Can you work these out from the model? Positions are in its coordinate system, mm. A direction names the side the tool comes from. Give positions to 0.01 mm unless a question says otherwise; leave off trailing zeros. Answer in a Markdown table with one row per item.
from build123d import *
from build123d.topology import SkipClean

# Parameters (mm, degrees)
SKETCH1_R           = 14.9
BOSS_EXTRUDE1_DEPTH = 2
SKETCH2_R           = 9.8
BOSS_EXTRUDE2_DEPTH = 8.5
SKETCH3_R           = 7.5
CUT_EXTRUDE1_DEPTH  = 5
THREAD1_PITCH       = 2
CUT_EXTRUDE2_START  = -3
SKETCH7_R           = 7.5
CUT_EXTRUDE2_DEPTH  = 3
SKETCH9_W           = 3.4
SKETCH9_H           = 17.333603835
BOSS_EXTRUDE3_DEPTH = 3
SKETCH10_R          = 0.75


with BuildPart() as part:
    # Sketch1 → Boss-Extrude1 (new body)
    with BuildSketch(Plane(origin=(0, 0, 0), x_dir=(1, 0, 0), z_dir=(0, 1, 0))):
        with Locations(Location((0, 0, 0), (0, 0, 270))):
            Circle(SKETCH1_R)
    extrude(amount=BOSS_EXTRUDE1_DEPTH)

    # Sketch2 → Boss-Extrude2 (add)
    with BuildSketch(Plane(origin=(0, 2, 0), x_dir=(1, 0, 0), z_dir=(0, 1, 0))):
        with Locations(Location((0, 0, 0), (0, 0, 270))):
            Circle(SKETCH2_R)
    extrude(amount=BOSS_EXTRUDE2_DEPTH)

    # Sketch3 → Cut-Extrude1 (cut)
    with BuildSketch(Plane(origin=(0, 10.5, 0), x_dir=(1, 0, 0), z_dir=(0, 1, 0))):
        with Locations(Location((0, 0, 0), (0, 0, 270))):
            Circle(SKETCH3_R)
    extrude(amount=-CUT_EXTRUDE1_DEPTH, mode=Mode.SUBTRACT)

    # Thread1: the profile of Sketch5 profile screwed along a right-hand helix of 5 turns, 10 arcs to a turn; built about Z, then put on its axis
    with SkipClean():  # the faces are left unmerged after this step: merging them gives an invalid solid
        thread1_z = Axis((0, 0, 0), (0, 0, 1))
        thread1_corners = [(9.8003, 0, -0.000173205), (9.8003, 0, 1.7501732), (8.71746825, 0, 1.124999997), (8.71746825, 0, 0.624999997)]
        with BuildLine(mode=Mode.PRIVATE) as thread1_profile:
            Line(thread1_corners[0], thread1_corners[1])
            Line(thread1_corners[1], thread1_corners[2])
            Line(thread1_corners[2], thread1_corners[3])
            Line(thread1_corners[3], thread1_corners[0])
        thread1_cap = Face(thread1_profile.wire())
        thread1_turn_angles = [0, 18, 36, 54, 72, 90, 108, 126, 144, 162, 180, 198, 216, 234, 252, 270, 288, 306, 324, 342, 360]
        thread1_turn_weights = [1, 0.9510565162951535, 1, 0.9510565162951535, 1, 0.9510565162951535, 1, 0.9510565162951535, 1, 0.9510565162951535, 1, 0.9510565162951535, 1, 0.9510565162951535, 1, 0.9510565162951535, 1, 0.9510565162951535, 1, 0.9510565162951535, 1]
        thread1_turn_rails = [Edge.make_bspline([Vector(p[0], p[1], 0).rotate(thread1_z, thread1_turn_angles[k]) / thread1_turn_weights[k] + Vector(0, 0, p[2] + THREAD1_PITCH * thread1_turn_angles[k] / 360) for k in range(21)], [0, 0, 0, 1, 1, 2, 2, 3, 3, 4, 4, 5, 5, 6, 6, 7, 7, 8, 8, 9, 9, 10, 10, 10], 2, thread1_turn_weights) for p in thread1_corners]
        thread1_turn_sides = [Face.make_surface_from_curves(thread1_turn_rails[p[0]], thread1_turn_rails[p[1]]) for p in [(0, 1), (1, 2), (2, 3), (3, 0)]]
        thread1 = Plane(origin=(0, 2, 0), x_dir=(1, 0, 0), z_dir=(0, 1, 0)) * Solid(Shell([*[p.moved(Location((0, 0, THREAD1_PITCH * i))) for i in range(5) for p in thread1_turn_sides], thread1_cap, thread1_cap.rotate(thread1_z, 1800).moved(Location((0, 0, THREAD1_PITCH * 1800 / 360)))]))
        add(thread1, mode=Mode.SUBTRACT)

    # Sketch7 → Cut-Extrude2 (cut)
    with SkipClean():  # the faces are left unmerged after this step: merging them gives an invalid solid
        with BuildSketch(Plane.XZ.offset(CUT_EXTRUDE2_START)):
            with Locations(Location((0, 0, 0), (0, 0, 90))):
                Circle(SKETCH7_R)
        extrude(amount=CUT_EXTRUDE2_DEPTH, mode=Mode.SUBTRACT)

    # Sketch9 → Boss-Extrude3 (add)
    with SkipClean():  # the faces are left unmerged after this step: merging them gives an invalid solid
        with BuildSketch(Plane.XZ.offset(-3)):
            with Locations((0, -0.102687227)):
                Rectangle(SKETCH9_W, SKETCH9_H)
        extrude(amount=BOSS_EXTRUDE3_DEPTH)

    # Sketch10 → Revolve1 (revolve)
    with SkipClean():  # the faces are left unmerged after this step: merging them gives an invalid solid
        with BuildSketch(Plane.XY, mode=Mode.PRIVATE) as revolve1_sk:
            with Locations((13, 2)):
                Circle(SKETCH10_R)
        revolve(revolve1_sk.sketch.rotate(Axis((0, 0, 0), (0, 1, 0)), 90), axis=Axis((0, 0, 0), (0, 1, 0)))


solid = part.part
Q1. For pin 1 (1.5 mm diameter, centred on y = 8, z = 7, fed in from +X); pin 2 (1.2 mm diameter, centred on x = 9.5, y = 2.5, fed in from -Z); pin 3 (3.5 mm diameter, centred on y = 1.5, z = -3.5, fed in from -X), each with a flat end and sliding along its axis, tell me the tip position at first contact or that it passes through.
Checked values:
| item | result |
|---|---|
| pin 1 | stops at x = 7.52 |
| pin 2 | stops at z = -11.75 |
| pin 3 | stops at x = -14.8 |
Q2. On a 3-axis mill with a long thin cutter (end or side, diameter ignored), from which of +Z, -Z, +X, -X, +Y, -Y can I reach the whole of each face in a straight line? I mean faces 4 (the face through (-5, 10.5, -6)), 5 (the face through (4, 3, 0)), 6 (the face through (8, 2, -6)), 7 (the face through (9, 3, 0)). Say none if no direction works.
Checked values:
| item | result |
|---|---|
| face 4 | +Z, -Z, +X, -X, +Y |
| face 5 | -Y |
| face 6 | +Y |
| face 7 | none |
Q3. If I drill on line 1 (Y direction, x = 2.75, z = 9); line 2 (Y direction, x = -8.5, z = 11); line 3 (Z direction, x = 2.25, y = 2.5), over which ranges is the centre line in solid material (lowest first)? Write a range as [from, to].
Checked values:
| item | result |
|---|---|
| line 1 | y = [0, 3.82], [5.12, 5.82], [7.12, 7.82], [9.12, 9.82] |
| line 2 | y = [0, 2] |
| line 3 | z = [-13.37, -12.24], [-9.4, -7.15], [7.15, 9.54], [12.24, 13.37] |
Q4. If we mould it in two halves opening along Z, with no side actions, what happens to faces 1 (the face through (-10, 2, 10)), 2 (the face through (-4, 3, 0)), 3 (the face through (-13.219, 0.986, 6.875))? For each: released by +Z, released by -Z, zero draft, split by the parting line, or undercut.
Checked values:
| item | result |
|---|---|
| face 1 | zero draft |
| face 2 | undercut |
| face 3 | split by the parting line |
